```python
from build123d import *

# Parameters (mm, degrees)
SKETCH147_W      = 3
SKETCH147_H      = 38.397224
EXTRUDE135_DEPTH = 7
SKETCH155_W      = 172
SKETCH155_H      = 37
EXTRUDE141_DEPTH = 3
SKETCH157_W      = 24
SKETCH157_H      = 21.68
EXTRUDE143_DEPTH = 4
SKETCH135_R      = 6.25
EXTRUDE123_DEPTH = 5
SKETCH_W         = 2
SKETCH_H         = 41.32


with BuildPart() as extrude135:
    # Sketch147 → Extrude135 (new body)
    with BuildSketch(Plane(origin=(0, 177, -3), x_dir=(1, 0, 0), z_dir=(0, -1, 0))):
        with Locations((345.5, -16.198612)):
            Rectangle(SKETCH147_W, SKETCH147_H)
    extrude(amount=-EXTRUDE135_DEPTH)


with BuildPart() as clamshell001:
    # Sketch155 → Extrude141 (new body)
    with BuildSketch(Plane.XY.offset(5.32)):
        with Locations((278, 287.5)):
            Rectangle(SKETCH155_W, SKETCH155_H)
    extrude(amount=EXTRUDE141_DEPTH)


with BuildPart() as extrude143:
    # Sketch157 → Extrude143 (new body)
    with BuildSketch(Plane(origin=(0, 304, 0), x_dir=(-1, 0, 0), z_dir=(0, 1, 0))):
        with Locations((-280, -26.16)):
            Rectangle(SKETCH157_W, SKETCH157_H)
    extrude(amount=EXTRUDE143_DEPTH)


with BuildPart() as clamshell002:
    # Sweep002: sweep along a path in Sketch166
    with BuildLine(Plane.XY.offset(6)) as sweep002_path:
        Line((192, 269), (192, 306))
        Line((192, 306), (364, 306))
        Line((364, 306), (364, 269))
    # Sketch165 → Sweep002 (sweep)
    with BuildSketch(Plane.YZ.offset(230)):
        Polygon((306.1, 5.32), (304.1, 3.32), (304.1, 8.32), (306.1, 8.32), align=None)
    sweep(path=sweep002_path.line, transition=Transition.RIGHT)


with BuildPart() as compound028:
    # Sketch135 → Extrude123 (new body)
    with BuildSketch(Plane.XZ.offset(-178)):
        with Locations((203, -14)):
            Circle(SKETCH135_R)
    extrude(amount=-EXTRUDE123_DEPTH)

    # Compound028: union Extrude135, clamshell001, Extrude143, clamshell002
    add(extrude135.part)
    add(clamshell001.part)
    add(extrude143.part)
    add(clamshell002.part)


with BuildPart() as walls:
    # Sweep: sweep along a path in Sketch133
    with BuildLine(Plane(origin=(0, 0, 5.32), x_dir=(1, 0, 0), z_dir=(0, 0, -1))) as sweep_path:
        Line((220.5, -182), (193, -182))
        Line((193, -182), (193, -305))
        Line((193, -305), (363, -305))
        Line((363, -305), (363, -182))
        Line((363, -182), (321.5, -182))
    # Sketch → Sweep (sweep)
    with BuildSketch(Plane(origin=(194, 0, 0), x_dir=(0, -1, 0), z_dir=(-1, 0, 0))):
        with Locations((-181, -13.34)):
            Rectangle(SKETCH_W, SKETCH_H)
    sweep(path=sweep_path.line, transition=Transition.RIGHT)

    # Cut: cut Compound028
    add(compound028.part, mode=Mode.SUBTRACT)


solid = walls.part
```
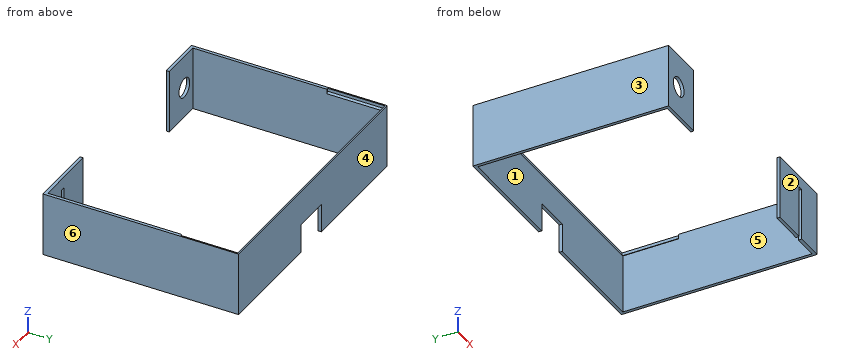
Could you check a few things on this model? Use its own coordinates, in mm. Face numbers are marked on the shaded views. A direction names the side the tool comes from. Give positions to 0.01 mm unless a question says otherwise; leave off trailing zeros. Order: outer loops, then holes, each group sorted by start corner. A loop starts at its lowest first (then second) coordinate and runs counter-clockwise, first axis right, second up.
Q1. Suppose I cut it at D-D, the plane x = 323.5. Write out the boundary of the cut face in (y, z), and give its area (3 significant figures).
Q2. Suppose I cut it at A-A, the plane y = 234.5. Write out the boundary of the cut face in (x, z).
Q3. We'd pull the mould along X, two halves only. Please class the marked faces 3, 4, 5 and 6: +X half, -X half, draft (parallel to the pull), parting line (faces both ways), or undercut.
Q4. For the marked faces 1 and 2, which set-ups out of +Z, -Z, +X, -X, +Y, -Y let a thin tool reach every point of the face, with its end or its side?
Q5. Suppose I cut it at C-C, the plane z = -23.5. Write out the boundary of the cut face in (x, y), and give its area (3 significant figures).
Q6. I'm going to push flat-ended pins straight in: P1, Ø2, axis at x = 277.5, y = 305.5, coming from the -Z side; P2, Ø0.6, axis at x = 303, z = 7, coming from the -Y side; P3, Ø8, axis at x = 281.5, z = 0, coming from the -Y side. Where does each tip first touch, or does it pass through?
Q7. If I drill on line 1 along Z through (x, y) = (203, 181.55); line 2 along X through (y, z) = (186.5, -6); line 3 along Y through (x, z) = (339, 0), over which ranges is the centre line in solid material (lowest first)?
Q8. Suppose I cut it at B-B, the plane x = 203. Write out the boundary of the cut face in (y, z), and give its area (3 significant figures).
Solution:
1. outline: (180, -34) - (182, -34) - (182, 7.32) - (180, 7.32) - close; (305, -34) - (307, -34) - (307, 7.32) - (306.1, 7.32) - (306.1, 5.32) - (305, 4.22) - close
1. area: 162 mm2
2. outline: (191, -34) - (193, -34) - (193, 7.32) - (191, 7.32) - close; (363, -34) - (365, -34) - (365, 7.32) - (363, 7.32) - close
3. face 3: -X half
3. face 4: draft
3. face 5: undercut
3. face 6: +X half
4. face 1: +Z, -Z
4. face 2: +Z, -Z, +X, -X, -Y
5. outline: (191, 180) - (220.5, 180) - (220.5, 182) - (193, 182) - (193, 305) - (268, 305) - (268, 307) - (191, 307) - close; (292, 305) - (363, 305) - (363, 182) - (347, 182) - (347, 180) - (365, 180) - (365, 307) - (292, 307) - close; (321.5, 180) - (344, 180) - (344, 182) - (321.5, 182) - close
5. area: 932 mm2
6. P1: stops at z = -15.32
6. P2: stops at y = 306.1
6. P3: stops at y = 305
7. line 1: z = -34 to -20.25, -7.75 to 7.32
7. line 2: x = 191 to 193, 363 to 365
7. line 3: y = 180 to 182, 305 to 307
8. outline: (180, -34) - (182, -34) - (182, -20.25) - (180, -20.25) - close; (180, -7.75) - (182, -7.75) - (182, 7.32) - (180, 7.32) - close; (305, -34) - (307, -34) - (307, 7.32) - (306.1, 7.32) - (306.1, 5.32) - (305, 4.22) - close
8. area: 137 mm2
